```python
from build123d import *

# Parameters (mm, degrees)
SKETCH1_W           = 27.305
SKETCH1_H           = 46.355
SKETCH1_W_2         = 22.225
SKETCH1_H_2         = 41.275
BOSS_EXTRUDE1_DEPTH = 6.35
SKETCH3_W           = 27.305
SKETCH3_H           = 46.355
BOSS_EXTRUDE2_DEPTH = 6.35
SKETCH4_R           = 1.397
CUT_EXTRUDE1_DEPTH  = 6.35


with BuildPart() as part:
    # Sketch1 → Boss-Extrude1 (new body)
    with BuildSketch(Plane(origin=(0, 0, 0), x_dir=(1, 0, 0), z_dir=(0, 1, 0))):
        with Locations((30.966827497, 1.604730882)):
            Rectangle(SKETCH1_W, SKETCH1_H)
        with Locations((30.966827497, 1.604730882)):
            Rectangle(SKETCH1_W_2, SKETCH1_H_2, mode=Mode.SUBTRACT)
    extrude(amount=-BOSS_EXTRUDE1_DEPTH)

    # Sketch3 → Boss-Extrude2 (add)
    with BuildSketch(Plane(origin=(0, -6.35, 0), x_dir=(-1, 0, 0), z_dir=(0, -1, 0))):
        with Locations((-30.966827497, 1.604730882)):
            Rectangle(SKETCH3_W, SKETCH3_H)
    extrude(amount=BOSS_EXTRUDE2_DEPTH)

    # Sketch4 → Cut-Extrude1 (cut)
    with BuildSketch(Plane(origin=(0, -6.35, 0), x_dir=(1, 0, 0), z_dir=(0, 1, 0))):
        with Locations(Location((39.395825841, 19.093107215, 0), (0, 0, 270))):
            Circle(SKETCH4_R)
        with Locations(Location((39.395865865, -15.704892785, 0), (0, 0, 270))):
            Circle(SKETCH4_R)
    extrude(amount=-CUT_EXTRUDE1_DEPTH, mode=Mode.SUBTRACT)


solid = part.part
```
Here's how the part is built. I have some questions about the finished solid (model axes, mm). A direction names the side the tool comes from. Give positions to 0.01 mm unless a question says otherwise; leave off trailing zeros. Write each loop counter-clockwise with the first axis right and the second up, starting at its lowest first coordinate (ties: lowest second). Pieces come first, ordered by that corner, then holes.
(1) Thinking about a two-plate mould opening in X: for faces 3 (the face through (17.314, -6, -1)), 4 (the face through (31, -6, -24.782)), 5 (the face through (42.079, -3, -1)), which applies, pulls with the +X half, pulls with the -X half, needs draft (parallel to the pull), parting line crosses it, or undercut?
Output values:
face 3: pulls with the -X half
face 4: needs draft
face 5: undercut
(2) Imagine slicing it at B-B, the plane x = 34.5. Write out the boundary of the cut face in (y, z).
Output values:
outline: (-12.7, -24.78) - (0, -24.78) - (0, -22.24) - (-6.35, -22.24) - (-6.35, 19.03) - (0, 19.03) - (0, 21.57) - (-12.7, 21.57) - close
(3) Imagine slicing it at D-D, the plane z = -8. Write out the boundary of the cut face in (x, y).
Output values:
outline: (17.31, -12.7) - (44.62, -12.7) - (44.62, 0) - (42.08, 0) - (42.08, -6.35) - (19.85, -6.35) - (19.85, 0) - (17.31, 0) - close
(4) Imagine slicing it at A-A, the plane y = -5.25. Write out the boundary of the cut face in (x, z), and give its area (3 significant figures).
Output values:
outline: (17.31, -24.78) - (44.62, -24.78) - (44.62, 21.57) - (17.31, 21.57) - close; hole (19.85, -22.24) - (42.08, -22.24) - (42.08, 19.03) - (19.85, 19.03) - close
area: 348 mm2
(5) If I drill on L1, parallel to Z at x = 35.75, y = -3.5; L2, parallel to X at y = -2.5, z = -1; L3, parallel to Y at x = 32.75, z = 6, over which ranges is the centre line in solid material (lowest first)?
Output values:
L1: z = -24.78 to -22.24, 19.03 to 21.57
L2: x = 17.31 to 19.85, 42.08 to 44.62
L3: y = -12.7 to -6.35
(6) Imagine slicing it at C-C, the plane x = 38.5. Write out the boundary of the cut face in (y, z).
Output values:
outline: (-12.7, -24.78) - (0, -24.78) - (0, -22.24) - (-6.35, -22.24) - (-6.35, -20.17) - (-12.7, -20.17) - close; (-12.7, -18.02) - (-6.35, -18.02) - (-6.35, 14.63) - (-12.7, 14.63) - close; (-12.7, 16.78) - (-6.35, 16.78) - (-6.35, 19.03) - (0, 19.03) - (0, 21.57) - (-12.7, 21.57) - close
(7) Will these pins go through, and if not, where does the flat tip stop? pin 1 (12 mm diameter, centred on x = 30, z = 4.5, fed in from +Y); pin 2 (2 mm diameter, centred on x = 20, z = -13, fed in from +Y).
Output values:
pin 1: stops at y = -6.35
pin 2: stops at y = 0
(8) On a 3-axis mill with a long thin cutter (end or side, diameter ignored), from which of +Z, -Z, +X, -X, +Y, -Y can I reach the whole of each face in a straight line? I mean faces 1 (the face through (31, -3, -22.242)), 2 (the face through (19, 0, -5)). Say none if no direction works.
Output values:
face 1: +Y
face 2: +Z, -Z, +X, -X, +Y
